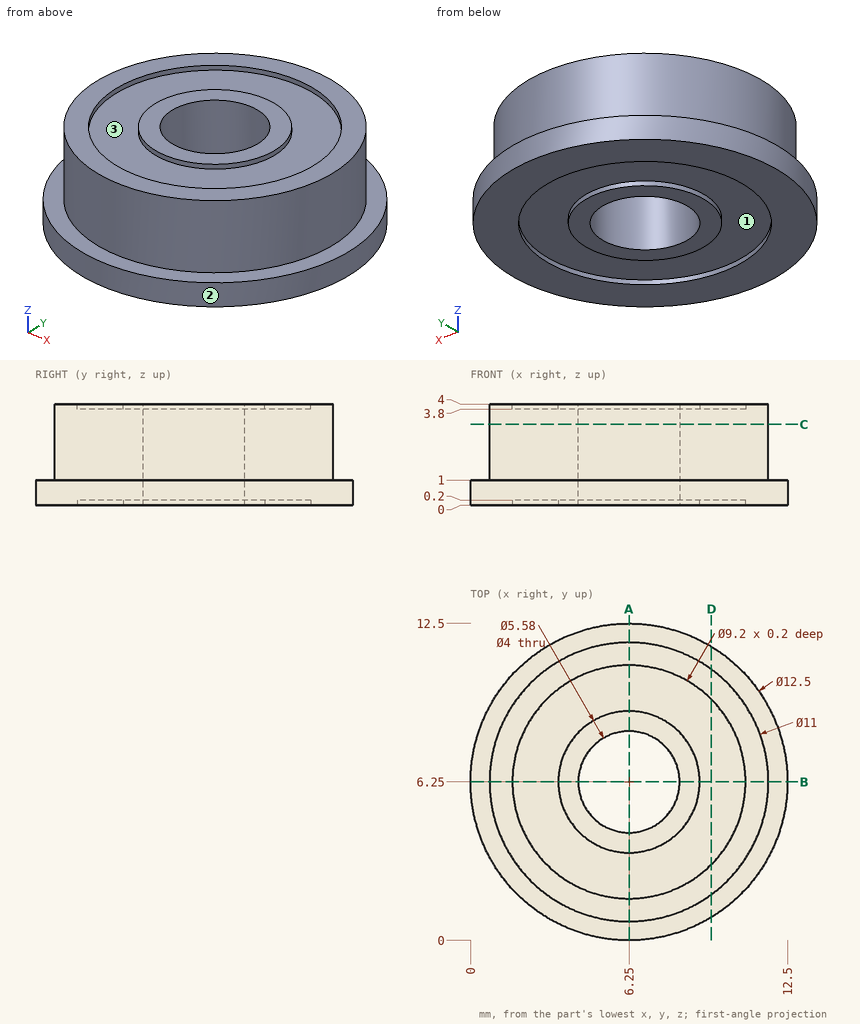
Design review of the part shown in the three views and the two pictorial views. Dimensions are in mm from the part's minimum x, y and z. A direction names the side the tool comes from. Round coordinates to 2 decimals unless told otherwise and drop trailing zeros. Order: outer loops, then holes, each group sorted by start corner. A loop starts at its lowest first (then second) coordinate and runs counter-clockwise, first axis right, second up.
(1) For P1, Ø1.5, axis at x = 3.5, z = 1, coming from the -Y side; P2, Ø1, axis at x = 3.5, z = 1, coming from the +Y side; P3, Ø1.5, axis at x = 2, z = 3, coming from the -Y side, all flat-tipped, find the tip position at first contact; note any pin that passes through.
Working result:
P1: stops at y = 0.33
P2: stops at y = 12.08
P3: stops at y = 2.01
(2) Take a section at D-D, the plane x = 9.5. State the section outline as (y, z) points.
Working result:
outline: (0.91, 0) - (2.99, 0) - (2.99, 0.2) - (9.51, 0.2) - (9.51, 0) - (11.59, 0) - (11.59, 1) - (10.69, 1) - (10.69, 4) - (9.51, 4) - (9.51, 3.8) - (2.99, 3.8) - (2.99, 4) - (1.81, 4) - (1.81, 1) - (0.91, 1) - close
(3) Take a section at C-C, the plane z = 3.2. State the section outline as (x, y) points.
Working result:
outline: circle Ø11 at (6.25, 6.25); hole circle Ø4 at (6.25, 6.25)
(4) Wall thickness on L1, parallel to Y at x = 6.25, z = 0.1; L2, parallel to Y at x = 6.25, z = 2.25; L3, parallel to Y at x = 6.25, z = 3.95: over which ranges is each line inside the solid? List them lowest first.
Working result:
L1: y = 0 to 1.65, 3.46 to 4.25, 8.25 to 9.04, 10.85 to 12.5
L2: y = 0.75 to 4.25, 8.25 to 11.75
L3: y = 0.75 to 1.65, 3.46 to 4.25, 8.25 to 9.04, 10.85 to 11.75
(5) Tool access review of the marked faces 1, 2 and 3: name each direction out of +Z, -Z, +X, -X, +Y, -Y from which nothing blocks a thin tool from reaching the whole face with its end or side.
Working result:
face 1: -Z
face 2: +Z, -Z
face 3: +Z
(6) Take a section at A-A, the plane x = 6.25. State the section outline as (y, z) points, plus the area to 3 significant figures.
Working result:
outline: (0, 0) - (1.65, 0) - (1.65, 0.2) - (3.46, 0.2) - (3.46, 0) - (4.25, 0) - (4.25, 4) - (3.46, 4) - (3.46, 3.8) - (1.65, 3.8) - (1.65, 4) - (0.75, 4) - (0.75, 1) - (0, 1) - close; (8.25, 0) - (9.04, 0) - (9.04, 0.2) - (10.85, 0.2) - (10.85, 0) - (12.5, 0) - (12.5, 1) - (11.75, 1) - (11.75, 4) - (10.85, 4) - (10.85, 3.8) - (9.04, 3.8) - (9.04, 4) - (8.25, 4) - close
area: 28.1 mm2
